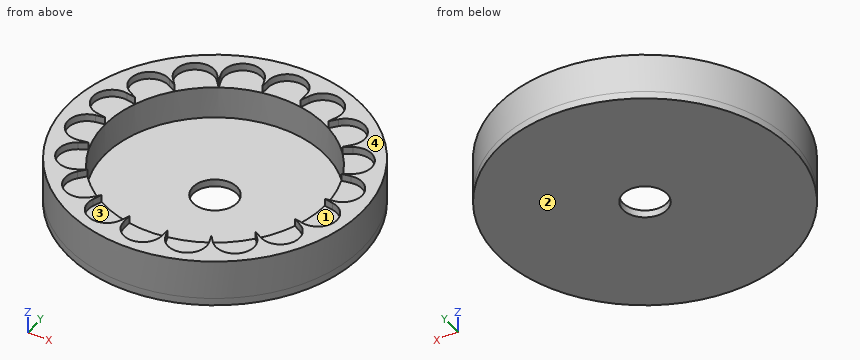
```python
from build123d import *

# Parameters (mm, degrees)
SKETCH1_R           = 63.5
SKETCH1_R_2         = 47.625
BOSS_EXTRUDE1_DEPTH = 17.018
CUT_EXTRUDE1_DEPTH  = 3.175
CIRPATTERN1_COUNT   = 10
CIRPATTERN1_ANGLE   = 180
BOSS_EXTRUDE2_START = 3.175
SKETCH3_R           = 63.5
SKETCH3_R_2         = 9.525
BOSS_EXTRUDE2_DEPTH = 3.175


with BuildPart() as part:
    # Sketch1 → Boss-Extrude1 (new body)
    with BuildSketch(Plane.XY):
        Circle(SKETCH1_R)
        Circle(SKETCH1_R_2, mode=Mode.SUBTRACT)
    extrude(amount=BOSS_EXTRUDE1_DEPTH)

    # Sketch2 → Cut-Extrude1 (cut)
    with BuildSketch(Plane.XY.offset(17.018)):
        with BuildLine():
            Line((8.255, 50.8), (8.255, -50.8))
            ThreePointArc((8.255, -50.8), (0, -59.055), (-8.255, -50.8))
            Line((-8.255, -50.8), (-8.255, 50.8))
            ThreePointArc((-8.255, 50.8), (0, 59.055), (8.255, 50.8))
        make_face()
    cut_extrude1 = extrude(amount=-CUT_EXTRUDE1_DEPTH, mode=Mode.SUBTRACT)

    # CirPattern1: Cut-Extrude1 ×10 about axis
    cirpattern1_axis = Axis((0, 0, 0), (0, 0, 1))
    for i in range(1, CIRPATTERN1_COUNT):
        add(cut_extrude1.rotate(cirpattern1_axis, i * CIRPATTERN1_ANGLE / (CIRPATTERN1_COUNT - 1)), mode=Mode.SUBTRACT)

    # Sketch3 → Boss-Extrude2 (add)
    with BuildSketch(Plane(origin=(0, 0, 0), x_dir=(-1, 0, 0), z_dir=(0, 0, -1)).offset(BOSS_EXTRUDE2_START)):
        Circle(SKETCH3_R)
        Circle(SKETCH3_R_2, mode=Mode.SUBTRACT)
    extrude(amount=-BOSS_EXTRUDE2_DEPTH)


solid = part.part
```
Build history of the part. All positions in model axes, mm. Face numbers are marked on the shaded views. A direction names the side the tool comes from. Give positions to 0.01 mm unless a question says otherwise; leave off trailing zeros. Order: outer loops, then holes, each group sorted by start corner. A loop starts at its lowest first (then second) coordinate and runs counter-clockwise, first axis right, second up. Notation, with made-up numbers: M 85,-35.75 L 134,-35.75 A28 ccw 134,-0.75 Z; hole C 66.5,74.25 d3. An arc over 180 degrees is marked long. Write item = value, one per line. Start each with the question number.
(1) Slice it at C-C on z = 2. Write the cut outline in (x, y) (3 decimals), plus the area to 3 significant figures.
(2) Pin check, flat tips, straight feed: pin 1 Ø10 at (y, z) = (6.5, 0.5) entering from -X; pin 2 Ø1.5 at (y, z) = (-32.5, 7) entering from +X; pin 3 Ø1 at (y, z) = (49.5, 15) entering from +X. Stop position of each tip, or through.
(3) Which spindle directions (+Z, -Z, +X, -X, +Y, -Y) get a long thin tool onto all of the face, cutting with end or side? Do the marked faces 1 and 2. Say none if no direction does.
(4) Slice it at B-B on y = -13.5. Write the cut outline in (x, z) (3 decimals), plus the area to 3 significant figures.
(5) Probe L1, parallel to X at y = 0, z = 9.5 (3 decimals); L2, parallel to Y at x = 0, z = -1.1 (3 decimals); L3, parallel to Y at x = -37.5, z = 16. List the from-to ranges inside material, lowest first. Write a range as [from, to].
(6) Two-plate mould, pull along Y, no slides. Class the marked faces 3 and 4: released by +Y, released by -Y, zero draft, split by the parting line, or undercut.
(7) Slice it at D-D on x = 29.5. Write the cut outline in (y, z) (3 decimals).
(8) Slice it at A-A on x = 0. Write the cut outline in (y, z) (3 decimals).
Responses:
q1.outline = C 0,0 d127; hole C 0,0 d95.25
q1.area = 5,540 mm2
q2.pin_1 = -63.48
q2.pin_2 = 54.99
q2.pin_3 = 40.39
q3.face_1 = +Z
q3.face_2 = -Z, +X, -X, +Y, -Y
q4.outline = M -62.048,-3.175 L 62.048,-3.175 L 62.048,17.018 L 56.829,17.018 L 56.829,13.843 L 45.672,13.843 L 45.672,0 L -45.672,0 L -45.672,13.843 L -56.829,13.843 L -56.829,17.018 L -62.048,17.018 Z
q4.area = 881 mm2
q5.L1 = [-63.5, -47.625], [47.625, 63.5]
q5.L2 = [-63.5, -9.525], [9.525, 63.5]
q5.L3 = [-51.24, -45.6], [-31.85, -31.18], [31.18, 31.85], [45.6, 51.24]
q6.face_3 = undercut
q6.face_4 = zero draft
q7.outline = M -56.232,-3.175 L 56.232,-3.175 L 56.232,17.018 L 46.544,17.018 L 46.544,13.843 L 37.388,13.843 L 37.388,0 L -37.388,0 L -37.388,13.843 L -46.544,13.843 L -46.544,17.018 L -56.232,17.018 Z
q8.outline = M -63.5,-3.175 L -9.525,-3.175 L -9.525,0 L -47.625,0 L -47.625,13.843 L -59.055,13.843 L -59.055,17.018 L -63.5,17.018 Z; M 9.525,-3.175 L 63.5,-3.175 L 63.5,17.018 L 59.055,17.018 L 59.055,13.843 L 47.625,13.843 L 47.625,0 L 9.525,0 Z
